The listing builds one solid part. Answer for the finished solid, in the listing's coordinates (mm). Face numbers are marked on the shaded views. A direction names the side the tool comes from. Give positions to 0.01 mm unless a question says otherwise; leave off trailing zeros. Write each loop counter-clockwise with the first axis right and the second up, starting at its lowest first coordinate (ties: lowest second). Pieces come first, ordered by that corner, then holes. Notation, with made-up numbers: M 3,22.5 L 7,22.5 A17 ccw 7,48.5 Z; hole C -15.75,69.25 d8. An arc over 180 degrees is marked long. Answer as a JSON object with one key per item and string values.
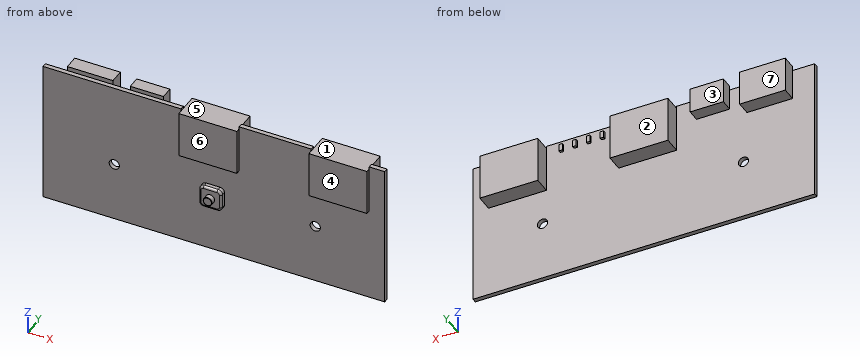
```python
from build123d import *

# Parameters (mm, degrees)
SKETCH1_W                = 77.2
SKETCH1_H                = 32.6
BOSS_EXTRUDE1_DEPTH      = 1
BOSS_EXTRUDE2_DEPTH      = 3.8
BOSS_EXTRUDE2_DEPTH_BACK = 2
SKETCH2_W                = 13.1
SKETCH2_H                = 11
SKETCH3_W                = 7.5
SKETCH3_H                = 5.7
BOSS_EXTRUDE3_DEPTH      = 2.8
SKETCH4_W                = 10.3
SKETCH4_H                = 8
BOSS_EXTRUDE4_DEPTH      = 3.2
SKETCH5_W                = 13.1
SKETCH5_H                = 5.8
CUT_EXTRUDE1_DEPTH       = 0.5
SKETCH6_W                = 0.8
SKETCH6_H                = 1.6
BOSS_EXTRUDE5_DEPTH      = 0.6
LPATTERN1_COUNT          = 4
LPATTERN1_PITCH          = 3.1
SKETCH7_W                = 5.1
SKETCH7_H                = 5.1
BOSS_EXTRUDE6_DEPTH      = 1.3
SKETCH8_R                = 1
BOSS_EXTRUDE7_DEPTH      = 1.2
FILLET1_R                = 1
FILLET2_R                = 0.5
FILLET3_R                = 0.1
SKETCH9_R                = 1.15
CUT_EXTRUDE2_DEPTH       = 43.469871674


with BuildPart() as part:
    # Sketch1 → Boss-Extrude1 (new body)
    with BuildSketch(Plane(origin=(0, 0, 0), x_dir=(1, 0, 0), z_dir=(0, 1, 0))):
        Rectangle(SKETCH1_W, SKETCH1_H)
    extrude(amount=BOSS_EXTRUDE1_DEPTH)

    # Sketch2 → Boss-Extrude2 (add, two sides: drawn at the far end of the back side and taken through both)
    with BuildSketch(Plane(origin=(0, 1, 0), x_dir=(1, 0, 0), z_dir=(0, 1, 0)).offset(-BOSS_EXTRUDE2_DEPTH_BACK)):
        with Locations((28.55, -10.8)):
            Rectangle(SKETCH2_W, SKETCH2_H)
        with Locations((-0.85, -10.8)):
            Rectangle(SKETCH2_W, SKETCH2_H)
    extrude(amount=BOSS_EXTRUDE2_DEPTH + BOSS_EXTRUDE2_DEPTH_BACK)

    # Sketch3 → Boss-Extrude3 (add)
    with BuildSketch(Plane(origin=(0, 1, 0), x_dir=(1, 0, 0), z_dir=(0, 1, 0))):
        with Locations((-15.65, -14.35)):
            Rectangle(SKETCH3_W, SKETCH3_H)
    extrude(amount=BOSS_EXTRUDE3_DEPTH)

    # Sketch4 → Boss-Extrude4 (add)
    with BuildSketch(Plane(origin=(0, 1, 0), x_dir=(1, 0, 0), z_dir=(0, 1, 0))):
        with Locations((-28.45, -13.3)):
            Rectangle(SKETCH4_W, SKETCH4_H)
    extrude(amount=BOSS_EXTRUDE4_DEPTH)

    # Sketch5 → Cut-Extrude1 (cut)
    with BuildSketch(Plane.XY.offset(16.3)):
        with Locations((-0.85, 1.9)):
            Rectangle(SKETCH5_W, SKETCH5_H)
        with Locations((28.55, 1.9)):
            Rectangle(SKETCH5_W, SKETCH5_H)
    extrude(amount=-CUT_EXTRUDE1_DEPTH, mode=Mode.SUBTRACT)

    # Sketch6 → Boss-Extrude5 (add)
    with BuildSketch(Plane(origin=(0, 1, 0), x_dir=(1, 0, 0), z_dir=(0, 1, 0))):
        with Locations((18.5, -14.5)):
            Rectangle(SKETCH6_W, SKETCH6_H)
    boss_extrude5 = extrude(amount=BOSS_EXTRUDE5_DEPTH)

    # LPattern1: Boss-Extrude5 ×4
    with Locations(*[(-i * LPATTERN1_PITCH, 0, 0) for i in range(1, LPATTERN1_COUNT)]):
        add(boss_extrude5)

    # Sketch7 → Boss-Extrude6 (add)
    with BuildSketch(Plane.XZ):
        with Locations((-0.15, -2.85)):
            Rectangle(SKETCH7_W, SKETCH7_H)
    extrude(amount=BOSS_EXTRUDE6_DEPTH)

    # Sketch8 → Boss-Extrude7 (add)
    with BuildSketch(Plane.XZ.offset(1.3)):
        with Locations(Location((-0.15, -2.85, 0), (0, 0, 90))):
            Circle(SKETCH8_R)
    extrude(amount=BOSS_EXTRUDE7_DEPTH)

    # Fillet1
    fillet1_edges = [part.edges().sort_by_distance(p)[0] for p in [
        (-2.7, -0.65, -0.3),
        (-2.7, -0.65, -5.4),
        (2.4, -0.65, -5.4),
        (2.4, -0.65, -0.3),
    ]]
    fillet(fillet1_edges, radius=FILLET1_R)

    # Fillet2
    fillet2_edges = [part.edges().sort_by_distance(p)[0] for p in [
        (-2.7, -1.3, -2.85),
        (-0.15, -1.3, -0.3),
        (-0.15, -1.3, -5.4),
        (2.4, -1.3, -2.85),
        (2.107106781, -1.3, -0.592893219),
        (-2.407106781, -1.3, -5.107106781),
        (2.107106781, -1.3, -5.107106781),
        (-2.407106781, -1.3, -0.592893219),
    ]]
    fillet(fillet2_edges, radius=FILLET2_R)

    # Fillet3
    fillet3_edges = [part.edges().sort_by_distance(p)[0] for p in [
        (-0.15, -2.5, -3.85),
    ]]
    fillet(fillet3_edges, radius=FILLET3_R)

    # Sketch9 → Cut-Extrude2 (cut, through all)
    with BuildSketch(Plane(origin=(0, 1, 0), x_dir=(1, 0, 0), z_dir=(0, 1, 0))):
        with Locations(Location((-22.5, 2.75, 0), (0, 0, 270))):
            Circle(SKETCH9_R)
        with Locations(Location((22.9, 2.75, 0), (0, 0, 270))):
            Circle(SKETCH9_R)
    extrude(amount=-CUT_EXTRUDE2_DEPTH, mode=Mode.SUBTRACT)


solid = part.part
```
1. Flat-ended cylindrical pins translate along their axes: pin 1 (4 mm diameter, centred on x = 2, y = 1.5, fed in from +Z); pin 2 (1 mm diameter, centred on y = 3, z = 11.5, fed in from -X); pin 3 (0.5 mm diameter, centred on y = -0.5, z = 9, fed in from +X). Find the tip coordinate at first contact, or state that the pin passes through.
Verdict:
{"pin 1": "stops at z = 15.8", "pin 2": "stops at x = -33.6", "pin 3": "stops at x = 35.1"}
2. The mould has two halves that part along X. Classify the marked faces 1 and 2: released by +X, released by -X, zero draft, split by the parting line, or undercut.
Verdict:
{"face 1": "undercut", "face 2": "zero draft"}
3. A cutting plane is placed at A-A, the plane x = 22.9. Give the vertices of the cut face in (y, z), plus the area to 3 significant figures.
Verdict:
{"outline": "M -1,5.3 L 0,5.3 L 0,-1.6 L 1,-1.6 L 1,5.3 L 4.8,5.3 L 4.8,15.8 L -1,15.8 Z; M 0,-16.3 L 1,-16.3 L 1,-3.9 L 0,-3.9 Z", "area": "80.2 mm2"}
4. A cutting plane is placed at C-C, the plane z = 8.5. Give the vertices of the cut face in (x, y).
Verdict:
{"outline": "M -38.6,0 L -7.4,0 L -7.4,-1 L 5.7,-1 L 5.7,0 L 22,0 L 22,-1 L 35.1,-1 L 35.1,0 L 38.6,0 L 38.6,1 L 35.1,1 L 35.1,4.8 L 22,4.8 L 22,1 L 5.7,1 L 5.7,4.8 L -7.4,4.8 L -7.4,1 L -38.6,1 Z"}
5. A cutting plane is placed at D-D, the plane z = -2.85. Give the vertices of the cut face in (x, y), plus the area to 3 significant figures.
Verdict:
{"outline": "M -38.6,0 L -23.65,0 L -23.65,1 L -38.6,1 Z; M -21.35,0 L -2.7,0 L -2.7,-0.8 A0.5 ccw -2.2,-1.3 L -1.15,-1.3 L -1.15,-2.4 A0.1 ccw -1.05,-2.5 L 0.75,-2.5 A0.1 ccw 0.85,-2.4 L 0.85,-1.3 L 1.9,-1.3 A0.5 ccw 2.4,-0.8 L 2.4,0 L 21.75,0 L 21.75,1 L -21.35,1 Z; M 24.05,0 L 38.6,0 L 38.6,1 L 24.05,1 Z", "area": "81.5 mm2"}
6. For the marked faces 3, 4, 5, 6 and 7, determine the directions among +Z, -Z, +X, -X, +Y, -Y from which every point of the face is accessible in a straight line to the end or side of a thin tool.
Verdict:
{"face 3": "+Z, -Z, +Y", "face 4": "+Z, -Z, +X, -X, -Y", "face 5": "+Z, +Y, -Y", "face 6": "+Z, +X, -X, -Y", "face 7": "+Z, -Z, -X, +Y"}
7. A cutting plane is placed at B-B, the plane y = 2.5. Give the vertices of the cut face in (x, z).
Verdict:
{"outline": "M -33.6,9.3 L -23.3,9.3 L -23.3,17.3 L -33.6,17.3 Z; M -19.4,11.5 L -11.9,11.5 L -11.9,17.2 L -19.4,17.2 Z; M -7.4,5.3 L 5.7,5.3 L 5.7,15.8 L -7.4,15.8 Z; M 22,5.3 L 35.1,5.3 L 35.1,15.8 L 22,15.8 Z"}
8. Consider line 1 along X through (y, z) = (0.8, -2.75); line 2 along X through (y, z) = (3.75, 12); line 3 along Z through (x, y) = (-3, 2.5). Determine where each line is inside the solid, lowest interval first.
Verdict:
{"line 1": "x = -38.6 to -23.65, -21.35 to 21.75, 24.05 to 38.6", "line 2": "x = -33.6 to -23.3, -19.4 to -11.9, -7.4 to 5.7, 22 to 35.1", "line 3": "z = 5.3 to 15.8"}
